Can you work these out from the model? Positions are in its coordinate system, mm. Face numbers are marked on the shaded views. A direction names the side the tool comes from. Give positions to 0.01 mm unless a question says otherwise; leave off trailing zeros. Write each loop counter-clockwise with the first axis right and the second up, starting at its lowest first coordinate (ties: lowest second). Pieces come first, ordered by that corner, then holes. Notation, with made-up numbers: (39, -20) -> (96, -20) arc R25 ccw to (96, 0) -> close; hole circle Ø6 at (18.25, 4.25). An arc over 180 degrees is marked (long way). Answer as CSV lines item,"result". Start each with the question number.
1. I need wall thicknesses on line 1 (Z direction, x = -29, y = 10); line 2 (Y direction, x = 10, z = 5); line 3 (X direction, y = 46, z = 10). Which ranges of each line are inside material? Lowest first, please. Write a range as [from, to].
2. If we section it at B-B on x = 0: Write out the boundary of the cut face in (y, z).
3. If we mould it in two halves opening along X, with no side actions, what happens to the marked faces 5, 6 and 7? For each: pulls with the +X half, pulls with the -X half, needs draft (parallel to the pull), parting line crosses it, or undercut.
4. If we section it at C-C on y = 0: Write out the boundary of the cut face in (x, z).
5. If we section it at D-D on y = -38: Write out the boundary of the cut face in (x, z).
6. I'm going to push flat-ended pins straight in: P1, Ø5, axis at x = 10, y = 33.5, coming from the +Z side; P2, Ø12.5, axis at x = 39, y = -8, coming from the +Z side; P3, Ø3, axis at x = 7, z = 8, coming from the -Y side; P4, Ø4, axis at y = -4, z = 9.5, coming from the -X side. Where does each tip first touch, or does it pass through?
7. If we section it at A-A on z = 10.5: Write out the boundary of the cut face in (x, y).
8. On a 3-axis mill with a long thin cutter (end or side, diameter ignored), from which of +Z, -Z, +X, -X, +Y, -Y can I reach the whole of each face in a straight line? I mean the marked faces 1, 2, 3 and 4. Say none if no direction works.
```python
from build123d import *

# Parameters (mm, degrees)
F0_R        = 51.5
F1_DEPTH    = 3
F2_W        = 44
F2_H        = 93.1289428696
F3_DEPTH    = 10
F5_DEPTH    = 93.1289428696
F6_T4_DEPTH = 93.1289428696
F6_S5_R     = 51.5
F6_T6_DEPTH = 48
F7_T4_DEPTH = 93.1289428696
F7_S5_R     = 51.5
F7_T6_DEPTH = 48


# Not quite as in the source:
# - a fillet or chamfer that OpenCascade refuses, or shapes differently, is made with other operations: its cross-section is extruded or revolved along the edge and cut away or added


with BuildPart() as f1:
    # F0 (on Top) → F1 (new body)
    with BuildSketch(Plane.XY):
        Circle(F0_R)
    extrude(amount=F1_DEPTH)

    # F2 (on face) → F3 (join)
    with BuildSketch(Plane.XY.offset(3)):
        Rectangle(F2_W, F2_H)
    extrude(amount=F3_DEPTH)

    # F4 (on face) → F5 (cut, through all)
    with BuildSketch(Plane(origin=(0, 46.5644714348, 0), x_dir=(-1, 0, 0), z_dir=(0, 1, 0))):
        with BuildLine():
            Line((17.6139149538, 13), (-17.6139149538, 13))
            ThreePointArc((-17.6139149538, 13), (0, 4.5), (17.6139149538, 13))
        make_face()
    extrude(amount=-F5_DEPTH, mode=Mode.SUBTRACT)

    # F6: fillet of radius 5 on 1 edges, made by hand


with BuildPart() as f6_tool2:
    # F6_s3 → F6_t4 (new body)
    with BuildSketch(Plane.XZ.offset(-46.5644714348)):
        with BuildLine():
            ThreePointArc((-27, 3), (-23.4644660941, 4.4644660941), (-22, 8))
            Line((-22, 8), (-22, 3))
            Line((-22, 3), (-27, 3))
        make_face()
    extrude(amount=F6_T4_DEPTH)

    # F6_s5 → F6_t6 (intersect, symmetric)
    with BuildSketch(Plane.XY.offset(5.5)):
        Circle(F6_S5_R)
    extrude(amount=F6_T6_DEPTH, both=True, mode=Mode.INTERSECT)


with BuildPart() as f1_1:
    add(f1.part)

    # F6_t1: union F6_tool2
    add(f6_tool2.part)

    # F7: fillet of radius 5 on 1 edges, made by hand


with BuildPart() as f7_tool2:
    # F7_s3 → F7_t4 (new body)
    with BuildSketch(Plane.XZ.offset(46.5644714348)):
        with BuildLine():
            ThreePointArc((27, 3), (23.4644660941, 4.4644660941), (22, 8))
            Line((22, 8), (22, 3))
            Line((22, 3), (27, 3))
        make_face()
    extrude(amount=-F7_T4_DEPTH)

    # F7_s5 → F7_t6 (intersect, symmetric)
    with BuildSketch(Plane.XY.offset(5.5)):
        Circle(F7_S5_R)
    extrude(amount=F7_T6_DEPTH, both=True, mode=Mode.INTERSECT)


with BuildPart() as f1_2:
    add(f1_1.part)

    # F7_t1: union F7_tool2
    add(f7_tool2.part)


solid = f1_2.part
```
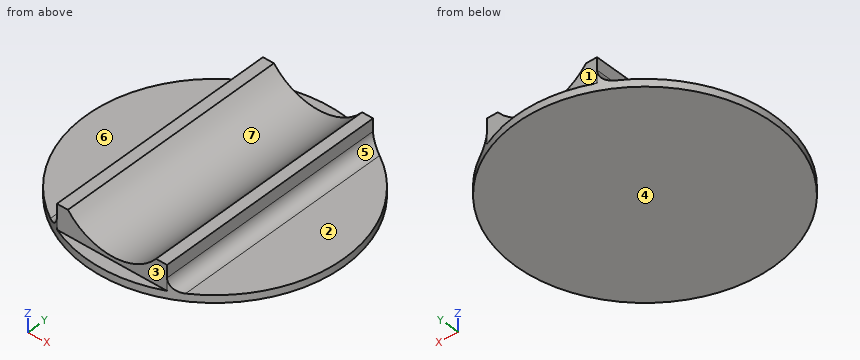
Computed values:
1,line 1,"z = [0, 3]"
1,line 2,"y = [-46.56, 46.56]"
1,line 3,"x = [-22, -14.74], [14.74, 22]"
2,outline,"(-51.5, 0) -> (51.5, 0) -> (51.5, 3) -> (46.56, 3) -> (46.56, 4.5) -> (-46.56, 4.5) -> (-46.56, 3) -> (-51.5, 3) -> close"
3,face 5,"pulls with the +X half"
3,face 6,"needs draft"
3,face 7,"undercut"
4,outline,"(-51.5, 0) -> (51.5, 0) -> (51.5, 3) -> (27, 3) arc R5 cw to (22, 8) -> (22, 13) -> (17.61, 13) arc R22.5 cw to (-17.61, 13) -> (-22, 13) -> (-22, 8) arc R5 cw to (-27, 3) -> (-51.5, 3) -> close"
5,outline,"(-34.76, 0) -> (34.76, 0) -> (34.76, 3) -> (27, 3) arc R5 cw to (22, 8) -> (22, 13) -> (17.61, 13) arc R22.5 cw to (-17.61, 13) -> (-22, 13) -> (-22, 8) arc R5 cw to (-27, 3) -> (-34.76, 3) -> close"
6,P1,"stops at z = 8.29"
6,P2,"stops at z = 3"
6,P3,"passes through"
6,P4,"stops at x = -22.03"
7,outline,"(-22, -46.56) -> (-15.3, -46.56) -> (-15.3, 46.56) -> (-22, 46.56) -> close; (15.3, -46.56) -> (22, -46.56) -> (22, 46.56) -> (15.3, 46.56) -> close"
8,face 1,"+Z, +X, -X, +Y"
8,face 2,"+Z, +X, +Y, -Y"
8,face 3,"+Z, +X, -X, -Y"
8,face 4,"-Z, +X, -X, +Y, -Y"
